```python
from build123d import *

# Parameters (mm, degrees)
SKETCH_1_R      = 1.5
EXTRUDE_1_DEPTH = 1.5
EXTRUDE_2_DEPTH = 5.5
SKETCH_3_W      = 8
SKETCH_3_H      = 10
EXTRUDE_3_DEPTH = 5
EXTRUDE_4_DEPTH = 10.000003


with BuildPart() as part:
    # Эскиз1 → Бобышка-Вытянуть1 (new body)
    with BuildSketch(Plane(origin=(0, 0, 0), x_dir=(1, 0, 0), z_dir=(0, 1, 0))):
        with BuildLine():
            Line((-28.198313686, 2.834587413), (-28.198313686, -13.165412587))
            ThreePointArc((-28.198313686, -13.165412587), (-27.31963403, -15.286732931), (-25.198313686, -16.165412587))
            Line((-25.198313686, -16.165412587), (-1.198313686, -16.165412587))
            ThreePointArc((-1.198313686, -16.165412587), (0.923006657, -15.286732931), (1.801686314, -13.165412587))
            Line((1.801686314, -13.165412587), (1.801686314, 2.834587413))
            ThreePointArc((1.801686314, 2.834587413), (0.923006657, 4.955907756), (-1.198313686, 5.834587413))
            Line((-1.198313686, 5.834587413), (-25.198313686, 5.834587413))
            ThreePointArc((-25.198313686, 5.834587413), (-27.31963403, 4.955907756), (-28.198313686, 2.834587413))
        make_face()
        with Locations(Location((-25.198313686, -13.165412587, 0), (0, 0, 270))):
            Circle(SKETCH_1_R, mode=Mode.SUBTRACT)
        with Locations(Location((-25.198313686, 2.834587413, 0), (0, 0, 270))):
            Circle(SKETCH_1_R, mode=Mode.SUBTRACT)
    extrude(amount=EXTRUDE_1_DEPTH)

    # Эскиз2 → Бобышка-Вытянуть2 (add)
    with BuildSketch(Plane(origin=(0, 1.5, 0), x_dir=(1, 0, 0), z_dir=(0, 1, 0))):
        Polygon((1.801686314, -0.165412587), (-6.698313686, -0.165412587), (-6.698313686, -10.165412587), (1.801686314, -10.165412587), (3.801686314, -10.165412587), (3.801686314, -0.165412587), align=None)
    extrude(amount=EXTRUDE_2_DEPTH)

    # Эскиз3 → Бобышка-Вытянуть3 (add)
    with BuildSketch(Plane(origin=(0, 1.5, 0), x_dir=(1, 0, 0), z_dir=(0, 1, 0))):
        with Locations((-17.198313686, -5.165412587)):
            Rectangle(SKETCH_3_W, SKETCH_3_H)
    extrude(amount=EXTRUDE_3_DEPTH)

    # Эскиз4 → Бобышка-Вытянуть4 (add)
    with BuildSketch(Plane.XY.offset(10.165412587)):
        Polygon((-21.198313686, 6.5), (-17.198313686, 6.5), (-17.198313686, 11.5), (-19.698313686, 11.5), align=None)
        Polygon((-17.198313686, 11.5), (-17.198313686, 6.5), (-13.198313686, 6.5), (-14.698313686, 11.5), align=None)
    extrude(amount=-EXTRUDE_4_DEPTH)


solid = part.part
```
Work out the finished part from the listing and answer in its coordinate system (mm). A direction names the side the tool comes from. Coordinates: 2 decimals unless noted, no trailing zeros. Write each loop counter-clockwise with the first axis right and the second up, starting at its lowest first coordinate (ties: lowest second). Pieces come first, ordered by that corner, then holes.
Q1. A cutting plane is placed at A-A, the plane y = 5.5. Give the vertices of the cut face in (x, z).
Q2. Each of these flat-tipped pins is pushed along its axis until it touches: pin 1 Ø0.6 at (x, z) = (2.5, 3.5) entering from -Y; pin 2 Ø6.5 at (x, y) = (-15.5, 7.5) entering from +Z; pin 3 Ø6 at (x, y) = (-11, 6.5) entering from -Z; pin 4 Ø4 at (x, z) = (-25.2, -2.83) entering from -Y. Where does it stop, or does it pass through?
Q3. Find the intervals of material crossed by line 1 (X direction, y = 4.25, z = 10); line 2 (Y direction, x = -11.5, z = 6.75); line 3 (X direction, y = 1.25, z = 6), in increasing order.
Q4. Determine the mould class of faces 1 (the face through (-28.198, 1, 5)), 2 (the face through (-17, 7, 10.165)), 3 (the face through (0.95, 0.74, -4.93)), 4 (the face through (-6.698, 4, 5)) for opening direction X: released by +X, released by -X, zero draft, split by the parting line, or undercut.
Q5. A cutting plane is placed at D-D, the plane z = -3.25. Give the vertices of the cut face in (x, y), then the cut area to 3 significant figures.
Q6. A cutting plane is placed at C-C, the plane z = 3. Give the vertices of the cut face in (x, y), then the cut area to 3 significant figures.
Q7. Which of the six approach directions +Z, -Z, +X, -X, +Y, -Y give full straight-line access (tool end or side, diameter ignored) to faces 5 (the face through (-21.198, 4, 5)), 6 (the face through (-13.198, 4, 5)), 7 (the face through (-17, 4, 0.165))?
Q8. A cutting plane is placed at B-B, the plane x = -5.5. Give the vertices of the cut face in (y, z).
Findings below:
1. outline: (-21.2, 0.17) - (-13.2, 0.17) - (-13.2, 10.17) - (-21.2, 10.17) - close; (-6.7, 0.17) - (3.8, 0.17) - (3.8, 10.17) - (-6.7, 10.17) - close
2. pin 1: stops at y = 1.5
2. pin 2: stops at z = 10.17
2. pin 3: stops at z = 0.17
2. pin 4: stops at y = 0
3. line 1: x = -21.2 to -13.2, -6.7 to 3.8
3. line 2: y = 0 to 1.5
3. line 3: x = -28.2 to 1.8
4. face 1: released by -X
4. face 2: zero draft
4. face 3: released by +X
4. face 4: undercut
5. outline: (-28.17, 0) - (-26.64, 0) - (-26.64, 1.5) - (-28.17, 1.5) - close; (-23.76, 0) - (1.77, 0) - (1.77, 1.5) - (-23.76, 1.5) - close
5. area: 40.6 mm2
6. outline: (-28.2, 0) - (1.8, 0) - (1.8, 1.5) - (3.8, 1.5) - (3.8, 7) - (-6.7, 7) - (-6.7, 1.5) - (-13.2, 1.5) - (-13.2, 6.5) - (-14.7, 11.5) - (-19.7, 11.5) - (-21.2, 6.5) - (-21.2, 1.5) - (-28.2, 1.5) - close
6. area: 175 mm2
7. face 5: +Z, -Z, -X, +Y
7. face 6: +Z, -Z, +Y
7. face 7: -Z, +X, -X, +Y
8. outline: (0, -5.83) - (1.5, -5.83) - (1.5, 0.17) - (7, 0.17) - (7, 10.17) - (1.5, 10.17) - (1.5, 16.17) - (0, 16.17) - close
